Autodesk Inventor part; units mm, degrees
ref_plane "РабПлоскость1" through (-2.9, -22, -69.5825) normal (-0.7071068, 0, -0.7071068) x (0, -1, 0)
ref_plane "YZ Plane" through (0, 0, 0) normal (1, 0, 0) x (0, 1, 0)
ref_plane "XZ Plane" through (0, 0, 0) normal (0, 1, 0) x (-1, 0, 0)
sketch "Эскиз1" plane through (0, 0, 0) normal (0, 1, 0) x (-1, 0, 0)
  arc A0 (-0.25, 9.2247) -> (0.25, 9.2247) centre (0, 8) ccw
  line L0 (-0.25, 10.9972) -> (-0.25, 9.2247)
  arc A1 (-0.25, 10.9972) -> (-1.1469, -10.94) centre (0, 0) ccw
  line L1 (-1.1469, -10.6297) -> (-1.1469, -10.94)
  line L2 (-0.8473, -10.6297) -> (-1.1469, -10.6297)
  line L3 (-0.8473, -10.9673) -> (-0.8473, -10.6297)
  arc A2 (-0.8473, -10.9673) -> (0.8535, -10.9668) centre (0, 0) ccw
  line L4 (0.8535, -10.6297) -> (0.8535, -10.9668)
  line L5 (1.1541, -10.6297) -> (0.8535, -10.6297)
  line L6 (1.1541, -10.9393) -> (1.1541, -10.6297)
  arc A3 (1.1541, -10.9393) -> (0.25, 10.9972) centre (0, 0) ccw
  line L7 (0.25, 9.2247) -> (0.25, 10.9972)
  circle A4 centre (8, 0) radius 1.25
  circle A5 centre (0, -8) radius 1.25
  circle A6 centre (-8, 0) radius 1.25
  circle A7 centre (0, -5.5) radius 0.75
  circle A8 centre (4.7631, 2.75) radius 0.75
  circle A9 centre (-4.7631, 2.75) radius 0.75
  circle A10 centre (0, 0) radius 2.9
  arc A11 (0.25, 9.2247) -> (-0.25, 9.2247) centre (0, 8) ccw
  circle A12 centre (0, 0) radius 11
extrude "Выдавливание1" add sketch "Эскиз1" along normal blind 22.76 contours A0 L7 A3 L6 L5 L4 A2 L3 L2 L1 A1 L0 | L0 A12 L7 A11 | L1 L2 L3 A12 | A12 L4 L5 L6
sketch "Эскиз2" plane through (0, 22.76, 0) normal (0, 1, 0) x (1, 0, 0)
  circle A0 centre (0, 0) radius 2.9
  line L0 (-2.9, 0) -> (2.9, 0)
  line L1 (2.9, 0) -> (2.9, 19.5825)
  line L2 (2.9, 19.5825) -> (-2.9, 19.5825)
  line L3 (-2.9, 19.5825) -> (-2.9, 0)
  circle A1 centre (0, 0) radius 11
  arc A2 (2.9, 10.6108) -> (-2.9, 10.6108) centre (0, 0) ccw
extrude "Выдавливание2" add sketch "Эскиз2" against normal blind 22.76 contours A1 L3 L2 L1
sketch "Эскиз3" plane through (0, 22.76, 0) normal (0, 1, 0) x (1, 0, 0)
  line L0 (2.9, 19.5825) -> (2.9, 10.6108)
  arc A0 (2.9, 10.6108) -> (-2.9, 10.6108) centre (0, 0) ccw
  line L1 (-2.9, 19.5825) -> (-2.9, 10.6108)
  line L2 (-2.9, 10.6108) -> (2.9, 10.6108)
  line L3 (2.9, 10.6108) -> (2.9, 19.5825)
  line L4 (2.9, 19.5825) -> (-2.9, 19.5825)
  line L5 (-2.9, 19.5825) -> (-2.9, 10.6108)
  point P0 (0, 0)
extrude "Выдавливание3" cut sketch "Эскиз3" against normal blind 1 contours L0 A0 L1 L4
sketch "Эскиз4" plane through (0, 0, 0) normal (0, -1, 0) x (1, 0, 0)
  arc A0 (-2.9, -10.6108) -> (2.9, -10.6108) centre (0, 0) ccw
  arc A1 (-2.9, -10.6108) -> (2.9, -10.6108) centre (0, 0) ccw
  line L0 (-2.9, -10.6108) -> (-2.9, -19.5825)
  line L1 (2.9, -10.6108) -> (-2.9, -10.6108)
  line L2 (-2.9, -10.6108) -> (-2.9, -19.5825)
  line L3 (-2.9, -19.5825) -> (2.9, -19.5825)
  line L4 (2.9, -19.5825) -> (2.9, -10.6108)
  point P0 (0, 0)
extrude "Выдавливание4" add sketch "Эскиз4" along normal blind 22 contours A0 L4 L3 L0
move faces "Перенос1" translate (0, 0, -50) faces at (-0.9667, 7.1733, -19.5825)
ref_plane "РабПлоскость1" through (-2.9, -22, -69.5825) normal (-0.7071068, 0, -0.7071068) x (0, -1, 0)
sketch "Эскиз5" plane through (-2.9, -22, -69.5825) normal (-0.7071068, 0, -0.7071068) x (0, -1, 0)
  line L0 (-43.76, 0) -> (0, 0)
  line L1 (-43.76, -4.1012) -> (-43.76, 37.598)
  line L2 (0, 0) -> (-43.76, 0)
  line L3 (-43.76, 0) -> (-43.76, -4.1012)
  line L4 (-43.76, -4.1012) -> (0, -4.1012)
  line L5 (0, -4.1012) -> (0, 0)
  point P0 (-22, 47.1516)
extrude "Выдавливание5" add sketch "Эскиз5" along normal blind 45 and the other way blind 4.25
properties part number "палец"
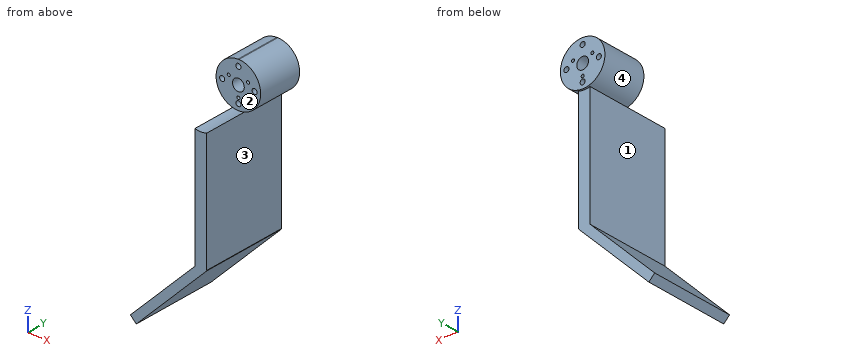
Geometry: final body of the model. Coordinates: model frame, mm. Face numbers are marked on the shaded views. A direction names the side the tool comes from. Round coordinates to 2 decimals unless told otherwise and drop trailing zeros. Order: outer loops, then holes, each group sorted by start corner. A loop starts at its lowest first (then second) coordinate and runs counter-clockwise, first axis right, second up.
Q1. Access query for the marked faces 3 and 4. Directions: +Z, -Z, +X, -X, +Y, -Y. A direction counts if a zero-diameter tool reaches every point of the face in a straight line with its end or side. Return the directions, or none.
Result sheet:
face 3: +X, +Y, -Y
face 4: -X, +Y, -Y
Q2. Material intervals for probe 1 along X at (y, z) = (7, 0); probe 2 along Z at (x, y) = (0, 7.75); probe 3 along Y at (x, z) = (-2.5, -3), sorted ascending.
Result sheet:
probe 1: x = -11 to -9.25, -6.75 to -2.9, 2.9 to 6.75, 9.25 to 11
probe 2: z = -72.48 to -9.25, -6.75 to -6.25, -4.75 to -2.9, 2.9 to 6.75, 9.25 to 11
probe 3: y = 0 to 22.76
Q3. Section B-B, the plane x = -8. Output: boundary loops of the cut face in (y, z).
Result sheet:
outline: (-22, -80.48) - (21.76, -80.48) - (21.76, -74.68) - (-22, -74.68) - close; (0, -7.55) - (22.76, -7.55) - (22.76, -1.25) - (0, -1.25) - close; (0, 1.25) - (22.76, 1.25) - (22.76, 7.55) - (0, 7.55) - close
Q4. Section D-D, the plane y = -6.5. Output: boundary loops of the cut face in (x, z).
Result sheet:
outline: (-34.72, -101.4) - (-31.82, -104.3) - (3.01, -69.48) - (2.9, -69.37) - (2.9, -10.61) arc R11 cw to (-2.9, -10.61) - (-2.9, -69.58) - close
Q5. Section A-A, the plane z = 0. Output: boundary loops of the cut face in (x, y), and give its area (3 significant figures).
Result sheet:
outline: (-11, 0) - (-9.25, 0) - (-9.25, 22.76) - (-11, 22.76) - close; (-6.75, 0) - (-2.9, 0) - (-2.9, 22.76) - (-6.75, 22.76) - close; (2.9, 0) - (6.75, 0) - (6.75, 22.76) - (2.9, 22.76) - close; (9.25, 0) - (11, 0) - (11, 22.76) - (9.25, 22.76) - close
area: 255 mm2
Q6. Section C-C, the plane y = 18. Give the number of separate pieces and of enclosed holes in the cut face, and give its area (3 significant figures).
Result sheet:
separate pieces: 1
enclosed holes: 8
area: 862 mm2
Q7. Mould query, pull axis Z, two halves, no side actions, for the marked faces 1 and 2. Classes: released by +Z, released by -Z, zero draft, split by the parting line, or undercut.
Result sheet:
face 1: undercut
face 2: zero draft
Q8. Pin query (flat end, axial travel): pin 1 (5 mm diameter, centred on y = 6, z = -14.5, fed in from -X); pin 2 (2 mm diameter, centred on x = -8, z = 0, fed in from -Y); pin 3 (4 mm diameter, centred on x = 0, z = 8, fed in from -Y); pin 4 (2 mm diameter, centred on y = 6, z = -5, fed in from -X). Return the tip coordinate at first contact, or that it passes through.
Result sheet:
pin 1: stops at x = -2.9
pin 2: passes through
pin 3: stops at y = 0
pin 4: stops at x = -10.25
